The listing builds one solid part. Answer for the finished solid, in the listing's coordinates (mm). Coordinates: 2 decimals unless noted, no trailing zeros. Order: outer loops, then holes, each group sorted by start corner. A loop starts at its lowest first (then second) coordinate and runs counter-clockwise, first axis right, second up. Notation, with made-up numbers: (15, -19.75) -> (24, -19.75) arc R14 cw to (24, 6.25) -> close; hole circle Ø7 at (-15, 34). An arc over 180 degrees is marked (long way). Return JSON: item names as keys, results as strings.
from build123d import *

# Parameters (mm, degrees)
SKETCH1_W               = 154
SKETCH1_H               = 304
BASE_FLANGE1_DEPTH      = 1
SKETCH4_W               = 22
SKETCH4_H               = 42
CUT_EXTRUDE3_DEPTH      = 10
MIRROR2_COPY_1_SKETCH_W = 22
MIRROR2_COPY_1_SKETCH_H = 42
MIRROR2_COPY_1_DEPTH    = 10
SKETCH2_R               = 2.05
CUT_EXTRUDE4_DEPTH      = 10


# Sheet-metal steps are written as plain solids
with BuildPart() as part:
    # Sketch1 → Base-Flange1 (new body)
    with BuildSketch(Plane(origin=(0, 0, 0), x_dir=(1, 0, 0), z_dir=(0, 1, 0))):
        with Locations((0, -117.655376963)):
            Rectangle(SKETCH1_W, SKETCH1_H)
    extrude(amount=-BASE_FLANGE1_DEPTH)

    # Sketch4 → Cut-Extrude3 (cut)
    with BuildSketch(Plane(origin=(0, 0, 0), x_dir=(1, 0, 0), z_dir=(0, 1, 0))):
        with Locations((0, -219.755376963)):
            Rectangle(SKETCH4_W, SKETCH4_H)
        with BuildLine():
            Line((-7.634176778, -205.755376963), (-7.634176778, -191.755376963))
            ThreePointArc((-7.634176778, -191.755376963), (-5.384176778, -189.505376963), (-3.134176778, -191.755376963))
            Line((-3.134176778, -191.755376963), (-3.134176778, -205.755376963))
            ThreePointArc((-3.134176778, -205.755376963), (-5.384176778, -208.005376963), (-7.634176778, -205.755376963))
        make_face()
    cut_extrude3 = extrude(amount=-CUT_EXTRUDE3_DEPTH, mode=Mode.SUBTRACT)

    # Mirror1: Cut-Extrude3 across plane
    add(cut_extrude3.mirror(Plane(origin=(0, 0, 0), x_dir=(0, 0, 1), z_dir=(1, 0, 0))), mode=Mode.SUBTRACT)

    # Mirror2: Cut-Extrude3 across plane
    add(cut_extrude3.mirror(Plane(origin=(0, 0, 219.755376963), x_dir=(1, 0, 0), z_dir=(0, 0, -1))), mode=Mode.SUBTRACT)

    # Mirror2 copy 1 sketch → Mirror2 copy 1 (cut)
    with BuildSketch(Plane(origin=(0, 0, 439.510753926), x_dir=(-1, 0, 0), z_dir=(0, 1, 0))):
        with Locations((0, -219.755376963)):
            Rectangle(MIRROR2_COPY_1_SKETCH_W, MIRROR2_COPY_1_SKETCH_H)
        with BuildLine():
            Line((-7.634176778, -205.755376963), (-7.634176778, -191.755376963))
            ThreePointArc((-7.634176778, -191.755376963), (-5.384176778, -189.505376963), (-3.134176778, -191.755376963))
            Line((-3.134176778, -191.755376963), (-3.134176778, -205.755376963))
            ThreePointArc((-3.134176778, -205.755376963), (-5.384176778, -208.005376963), (-7.634176778, -205.755376963))
        make_face()
    extrude(amount=-MIRROR2_COPY_1_DEPTH, mode=Mode.SUBTRACT)

    # Sketch2 → Cut-Extrude4 (cut)
    with BuildSketch(Plane(origin=(0, 0, 0), x_dir=(1, 0, 0), z_dir=(0, 1, 0))):
        with Locations(Location((-45.02, -263.475376963, 0), (0, 0, 270))):
            Circle(SKETCH2_R)
        with Locations(Location((-45.02, -173.435376963, 0), (0, 0, 270))):
            Circle(SKETCH2_R)
        with Locations(Location((45.02, -173.435376963, 0), (0, 0, 270))):
            Circle(SKETCH2_R)
        with Locations(Location((45.02, -263.475376963, 0), (0, 0, 270))):
            Circle(SKETCH2_R)
    extrude(amount=-CUT_EXTRUDE4_DEPTH, mode=Mode.SUBTRACT)


solid = part.part
1. The part is cut by section B-B on y = -0.55. Give the vertices of the cut face in (x, z), and give its area (3 significant figures).
Answer block:
{"outline": "(-77, -34.34) -> (77, -34.34) -> (77, 269.66) -> (-77, 269.66) -> close; hole circle Ø4.1 at (-45.02, 173.44); hole circle Ø4.1 at (-45.02, 263.48); hole (-11, 198.76) -> (-7.63, 198.76) -> (-7.63, 191.76) arc R2.25 ccw to (-3.13, 191.76) -> (-3.13, 198.76) -> (3.13, 198.76) -> (3.13, 191.76) arc R2.25 ccw to (7.63, 191.76) -> (7.63, 198.76) -> (11, 198.76) -> (11, 240.76) -> (7.63, 240.76) -> (7.63, 247.76) arc R2.25 ccw to (3.13, 247.76) -> (3.13, 240.76) -> (-3.13, 240.76) -> (-3.13, 247.76) arc R2.25 ccw to (-7.63, 247.76) -> (-7.63, 240.76) -> (-11, 240.76) -> close; hole circle Ø4.1 at (45.02, 173.44); hole circle Ø4.1 at (45.02, 263.48)", "area": "45,700 mm2"}
2. This flat-tipped pin is pushed along its axis until it touches: pin 1 Ø3.5 at (x, z) = (-45.02, 173.44) entering from +Y. Where does it stop, or does it pass through?
Answer block:
{"pin 1": "passes through"}
3. Consider line 1 (X direction, y = -0.85, z = 245.5); line 2 (X direction, y = -0.45, z = 208); line 3 (Z direction, x = -10, y = -0.55). Determine where each line is inside the solid, lowest interval first. Write a range as from..to.
Answer block:
{"line 1": "x = -77..-7.63, -3.13..3.13, 7.63..77", "line 2": "x = -77..-11, 11..77", "line 3": "z = -34.34..198.76, 240.76..269.66"}
4. The part is cut by section A-A on z = 244. Give the vertices of the cut face in (x, y), and give its area (3 significant figures).
Answer block:
{"outline": "(-77, -1) -> (-7.63, -1) -> (-7.63, 0) -> (-77, 0) -> close; (-3.13, -1) -> (3.13, -1) -> (3.13, 0) -> (-3.13, 0) -> close; (7.63, -1) -> (77, -1) -> (77, 0) -> (7.63, 0) -> close", "area": "145 mm2"}
